Could you check a few things on this model? Use its own coordinates, in mm. Face numbers are marked on the shaded views. Coordinates: 2 decimals unless noted, no trailing zeros. Loops run counter-clockwise (first coordinate to the right, second up) from the corner with the lowest first, then second, coordinate; pieces in that order, holes last.
from build123d import *

# Parameters (mm, degrees)
SKETCH1_R                      = 35
BOSS_EXTRUDE1_DEPTH            = 40
SKETCH2_R                      = 16.25
CUT_EXTRUDE1_DEPTH             = 5
M4_CLEARANCE_HOLE1_D           = 4.5
M4_CLEARANCE_HOLE1_DEPTH       = 13
M4_CLEARANCE_HOLE1_CSINK_D     = 4.55
M4_CLEARANCE_HOLE1_CSINK_ANGLE = 90
M4_CLEARANCE_HOLE1_TIP         = 1.351936393
FILLET4_R                      = 10


with BuildPart() as part:
    # Sketch1 → Boss-Extrude1 (new body)
    with BuildSketch(Plane(origin=(0, 0, 0), x_dir=(1, 0, 0), z_dir=(0, 1, 0))):
        Circle(SKETCH1_R)
    extrude(amount=BOSS_EXTRUDE1_DEPTH)

    # Sketch2 → Cut-Extrude1 (cut)
    with BuildSketch(Plane(origin=(0, 40, 0), x_dir=(1, 0, 0), z_dir=(0, 1, 0))):
        Circle(SKETCH2_R)
    extrude(amount=-CUT_EXTRUDE1_DEPTH, mode=Mode.SUBTRACT)

    # M4 Clearance Hole1
    with Locations(Plane(origin=(0, 35, 0), x_dir=(1, 0, 0), z_dir=(0, 1, 0))):
        with Locations((-8, 8), (8, 8), (8, -8), (-8, -8)):
            CounterSinkHole(M4_CLEARANCE_HOLE1_D / 2, M4_CLEARANCE_HOLE1_CSINK_D / 2, depth=M4_CLEARANCE_HOLE1_DEPTH, counter_sink_angle=M4_CLEARANCE_HOLE1_CSINK_ANGLE)
            with Locations((0, 0, -(M4_CLEARANCE_HOLE1_DEPTH + M4_CLEARANCE_HOLE1_TIP / 2))):  # 118° drill point
                Cone(0, M4_CLEARANCE_HOLE1_D / 2, M4_CLEARANCE_HOLE1_TIP, mode=Mode.SUBTRACT)

    # Fillet4
    fillet4_edges = [part.edges().sort_by_distance(p)[0] for p in [
        (-35, 0, 0),
        (-35, 40, 0),
    ]]
    fillet(fillet4_edges, radius=FILLET4_R)


solid = part.part
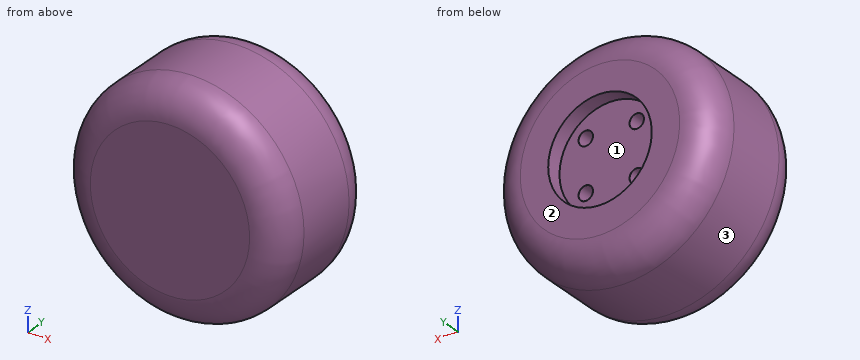
1) If I drill on L1, parallel to X at y = 22.5, z = 8; L2, parallel to Z at x = -15, y = 36; L3, parallel to Z at x = -8, y = 30.75, over which ranges is the centre line in solid material (lowest first)?
2) Imagine slicing it at D-D on y = 4.5. List the corners of the cut face in (x, z) for me, plus the area to 3 significant figures.
3) Imagine slicing it at C-C on z = 0. List the corners of the cut face in (x, y) for me, plus the area to 3 significant figures.
4) Imagine slicing it at B-B on y = 25. List the corners of the cut face in (x, z) for me.
5) We'd pull the mould along X, two halves only. Please class the marked faces 1, 2 and 3: released by +X, released by -X, zero draft, split by the parting line, or undercut.
6) Will these pins go through, and if not, where does the flat tip stop? pin 1 (4 mm diameter, centred on x = -16.5, y = 10, fed in from -Z); pin 2 (6 mm diameter, centred on x = 16.5, y = 5, fed in from -Z); pin 3 (10 mm diameter, centred on x = -3, z = 6.5, fed in from +Y).
7) Imagine slicing it at A-A on x = 0. List the corners of the cut face in (y, z) for me.
Solved:
1. L1: x = -34.07 to -10.25, -5.75 to 5.75, 10.25 to 34.07
1. L2: z = -29.39 to -6.25, 6.25 to 29.39
1. L3: z = -34.04 to -10.25, -5.75 to 5.75, 10.25 to 34.04
2. outline: circle Ø66.7 at (0, 0)
2. area: 3,490 mm2
3. outline: (-35, 10) arc R10 ccw to (-25, 0) - (25, 0) arc R10 ccw to (35, 10) - (35, 30) arc R10 ccw to (25, 40) - (16.25, 40) - (16.25, 35) - (-16.25, 35) - (-16.25, 40) - (-25, 40) arc R10 ccw to (-35, 30) - close
3. area: 2,550 mm2
4. outline: circle Ø70 at (0, 0); hole circle Ø4.5 at (-8, -8); hole circle Ø4.5 at (-8, 8); hole circle Ø4.5 at (8, -8); hole circle Ø4.5 at (8, 8)
5. face 1: undercut
5. face 2: zero draft
5. face 3: split by the parting line
6. pin 1: stops at z = -31.86
6. pin 2: stops at z = -31.46
6. pin 3: stops at y = 35
7. outline: (0, -25) arc R10 ccw to (10, -35) - (30, -35) arc R10 ccw to (40, -25) - (40, -16.25) - (35, -16.25) - (35, 16.25) - (40, 16.25) - (40, 25) arc R10 ccw to (30, 35) - (10, 35) arc R10 ccw to (0, 25) - close
